Verification items for the finished model (mm, model axes). A direction names the side the tool comes from. Coordinates: 2 decimals unless noted, no trailing zeros. Order: outer loops, then holes, each group sorted by start corner. A loop starts at its lowest first (then second) coordinate and runs counter-clockwise, first axis right, second up. Notation, with made-up numbers: M -7.5,-36 L 36.5,-36 A16 ccw 36.5,-17 Z; hole C -21.75,28.25 d3. An arc over 180 degrees is marked long. Return JSON: item names as keys, results as strings. Group by question number.
Q1. Section check A-A, the plane x = 175. Enter the section's corners in (y, z), then the cut area to 3 significant figures.
Q2. Go/stop test with flat-tipped pins: pin 1 Ø0.8 at (x, y) = (207.5, 42) entering from -Z; pin 2 Ø4 at (y, z) = (59.5, -37) entering from +X; pin 3 Ø1 at (y, z) = (103.5, -21) entering from -X. Record where each tip stops, or that it passes through.
Q3. Mould release check, pull along X, two halves, no side actions. Record for faces 1 (the face through (247.156, 72, -33)), 2 (the face through (209, 60, -27.181)), 3 (the face through (233.615, 72.507, -36.255)): pulls with the +X half, pulls with the -X half, needs draft (parallel to the pull), parting line crosses it, or undercut.
Q4. Access from +Z, -Z, +X, -X, +Y, -Y to the whole of each face (thin tool, end or side, straight path). Record for faces 4 (the face through (205.102, 71.014, -31.062)), 5 (the face through (209, 50, -41)), 6 (the face through (207, 3, -65)), 7 (the face through (203.757, 57, -27)).
Q5. Section check B-B, the plane y = 157. Enter the section's corners in (x, z), then the cut area to 3 significant figures.
Q6. Section check D-D, the plane y = 101. Enter the section's corners in (x, z), then the cut area to 3 significant figures.
Q7. Thickness scan on probe 1 along X at (y, z) = (70.75, -33); probe 2 along X at (y, z) = (47, -143); probe 3 along Y at (x, z) = (177.5, -110). Record the ranges inside material, lowest first.
Q8. Section check C-C, the plane z = -125. Enter the section's corners in (x, y).
from build123d import *

# Parameters (mm, degrees)
EXTRUDE_1_DEPTH     = 225
SKETCH_3_W          = 66
SKETCH_3_H          = 76.655878063
EXTRUDE_2_DEPTH     = 3
SKETCH_4_W          = 76.655878063
SKETCH_4_H          = 33
EXTRUDE_3_DEPTH     = 3
SKETCH_5_W          = 76.655878063
SKETCH_5_H          = 33
EXTRUDE_4_DEPTH     = 3
SKETCH_7_R          = 25
CUT_EXTRUDE_1_DEPTH = 1
SKETCH_8_R          = 4.2
CUT_EXTRUDE_2_DEPTH = 3
CUT_EXTRUDE_3_DEPTH = 3
SKETCH_10_W         = 6.167449304
SKETCH_10_H         = 10.561253057
EXTRUDE_5_DEPTH     = 20
SKETCH_11_W         = 10.561253057
SKETCH_11_H         = 34.261699871
EXTRUDE_6_DEPTH     = 3
EXTRUDE_7_DEPTH     = 3
EXTRUDE_8_DEPTH     = 43
SKETCH_15_W         = 76.655878063
SKETCH_15_H         = 2.5
EXTRUDE_9_DEPTH     = 3


with BuildPart() as part:
    # 草图1 → 凸台-拉伸1 (new body)
    with BuildSketch(Plane(origin=(0, 0, 0), x_dir=(1, 0, 0), z_dir=(0, 1, 0))):
        with BuildLine():
            Line((0, 0), (40, 0))
            ThreePointArc((40, 0), (100, 60), (160, 0))
            Line((160, 0), (170.5, 0))
            Line((170.5, 0), (170.5, 180))
            Line((170.5, 180), (168, 180))
            Line((168, 180), (168, 2.5))
            Line((168, 2.5), (162, 2.5))
            ThreePointArc((162, 2.5), (99.5, 62.720665032), (37, 2.5))
            Line((37, 2.5), (0, 2.5))
            Line((0, 2.5), (0, 0))
        make_face()
    extrude(amount=EXTRUDE_1_DEPTH)

    # 草图3 → 凸台-拉伸2 (add)
    with BuildSketch(Plane(origin=(0, 70, 0), x_dir=(0, 0, -1), z_dir=(0, -1, 0))):
        with Locations((33, 208.827939032)):
            Rectangle(SKETCH_3_W, SKETCH_3_H)
    extrude(amount=-EXTRUDE_2_DEPTH)

    # 草图4 → 凸台-拉伸3 (add)
    with BuildSketch(Plane.XY):
        with Locations((208.827939032, 89.5)):
            Rectangle(SKETCH_4_W, SKETCH_4_H)
    extrude(amount=-EXTRUDE_3_DEPTH)

    # 草图5 → 凸台-拉伸4 (add)
    with BuildSketch(Plane(origin=(0, 0, -66), x_dir=(-1, 0, 0), z_dir=(0, 0, -1))):
        with Locations((-208.827939032, 89.5)):
            Rectangle(SKETCH_5_W, SKETCH_5_H)
    extrude(amount=-EXTRUDE_4_DEPTH)

    # 草图7 → 切除-拉伸1 (cut)
    with BuildSketch(Plane(origin=(0, 73, 0), x_dir=(1, 0, 0), z_dir=(0, 1, 0))):
        with Locations(Location((208.827939031, 33, 0), (0, 0, 270))):
            Circle(SKETCH_7_R)
    extrude(amount=-CUT_EXTRUDE_1_DEPTH, mode=Mode.SUBTRACT)

    # 草图8 → 切除-拉伸2 (cut)
    with BuildSketch(Plane(origin=(0, 73, 0), x_dir=(1, 0, 0), z_dir=(0, 1, 0))):
        with Locations(Location((208.827939031, 33, 0), (0, 0, 270))):
            Circle(SKETCH_8_R)
    extrude(amount=-CUT_EXTRUDE_2_DEPTH, mode=Mode.SUBTRACT)

    # 草图9 → 切除-拉伸3 (cut)
    with BuildSketch(Plane(origin=(0, 73, 0), x_dir=(1, 0, 0), z_dir=(0, 1, 0))):
        with BuildLine():
            Line((202.276441695, 38.603794928), (202.276441695, 54.71078199))
            ThreePointArc((202.276441695, 54.71078199), (187.355723059, 33.535648138), (202.276441695, 12.360514285))
            Line((202.276441695, 12.360514285), (202.276441695, 26.245847959))
            Line((202.276441695, 26.245847959), (202.276441695, 38.603794928))
        make_face()
        with BuildLine():
            ThreePointArc((215.331215104, 54.71078199), (229.726697753, 33.535648138), (215.331215104, 12.360514285))
            Line((215.331215104, 12.360514285), (215.331215104, 26.245847959))
            Line((215.331215104, 26.245847959), (215.331215104, 38.603794928))
            Line((215.331215104, 38.603794928), (215.331215104, 54.71078199))
        make_face()
    extrude(amount=-CUT_EXTRUDE_3_DEPTH, mode=Mode.SUBTRACT)

    # 草图10 → 凸台-拉伸5 (add)
    with BuildSketch(Plane(origin=(0, 70, 0), x_dir=(0, 0, -1), z_dir=(0, -1, 0))):
        with Locations((24.097577195, 209.037691234)):
            Rectangle(SKETCH_10_W, SKETCH_10_H)
    extrude(amount=EXTRUDE_5_DEPTH)

    # 草图11 → 凸台-拉伸6 (add)
    with BuildSketch(Plane(origin=(0, 50, 0), x_dir=(-1, 0, 0), z_dir=(0, -1, 0))):
        with Locations((-209.037691234, 38.144702479)):
            Rectangle(SKETCH_11_W, SKETCH_11_H)
    extrude(amount=EXTRUDE_6_DEPTH)

    # 草图12 → 凸台-拉伸7 (add)
    with BuildSketch(Plane(origin=(0, 0, 0), x_dir=(1, 0, 0), z_dir=(0, 1, 0))):
        Polygon((170.5, 0), (247.155878063, 0), (247.205159598, 131.685407984), (170.5, 131.685407984), align=None)
    extrude(amount=EXTRUDE_7_DEPTH)

    # 草图13 → 凸台-拉伸8 (add)
    with BuildSketch(Plane(origin=(0, 0, 0), x_dir=(1, 0, 0), z_dir=(0, 1, 0))):
        Polygon((247.155878063, 0), (247.205159598, 131.685407984), (170.5, 131.685407984), (170.5, 129.185407984), (244.763652704, 129.185407984), (244.763652704, 0), align=None)
    extrude(amount=EXTRUDE_8_DEPTH)

    # 草图15 → 凸台-拉伸9 (add)
    with BuildSketch(Plane.XY):
        with Locations((208.827939032, 41.75)):
            Rectangle(SKETCH_15_W, SKETCH_15_H)
    extrude(amount=-EXTRUDE_9_DEPTH)


solid = part.part
Numbers:
{
 "1": {"outline": "M 0,-131.69 L 43,-131.69 L 43,-129.19 L 3,-129.19 L 3,0 L 0,0 Z; M 40.5,-3 L 43,-3 L 43,0 L 40.5,0 Z; M 70,-66 L 106,-66 L 106,-63 L 73,-63 L 73,-3 L 106,-3 L 106,0 L 70,0 Z", "area": "899 mm2"},
 "2": {"pin 1": "stops at z = -131.69", "pin 2": "stops at x = 170.5", "pin 3": "stops at x = 40.35"},
 "3": {"face 1": "pulls with the +X half", "face 2": "needs draft", "face 3": "undercut"},
 "4": {"face 4": "+Y", "face 5": "-Z, +X", "face 6": "+Z", "face 7": "+Z, -Z"},
 "5": {"outline": "M 0,-2.5 L 37,-2.5 A62.54 ccw 162,-2.5 L 168,-2.5 L 168,-180 L 170.5,-180 L 170.5,0 L 160,0 A60 cw 40,0 L 0,0 Z", "area": "1,070 mm2"},
 "6": {"outline": "M 0,-2.5 L 37,-2.5 A62.54 ccw 162,-2.5 L 168,-2.5 L 168,-180 L 170.5,-180 L 170.5,-66 L 247.16,-66 L 247.16,-63 L 170.5,-63 L 170.5,-3 L 247.16,-3 L 247.16,0 L 160,0 A60 cw 40,0 L 0,0 Z", "area": "1,530 mm2"},
 "7": {"probe 1": "x = 46.26 to 49.89, 150.11 to 152.74, 168 to 187.36, 202.28 to 204.63, 213.03 to 215.33, 229.72 to 247.16", "probe 2": "x = 168 to 170.5", "probe 3": "y = 0 to 3"},
 "8": {"outline": "M 168,0 L 247.2,0 L 247.2,43 L 244.76,43 L 244.76,3 L 170.5,3 L 170.5,225 L 168,225 Z"}
}
